from build123d import *

# Parameters (mm, degrees)
Y_KSEKLIK_EKSTR_ZYON1_DEPTH = 3.2
IZIM2_OUTSIDE_W             = 23.4
IZIM2_OUTSIDE_H             = 22.318
IZIM2_OUTSIDE_R             = 3.5
KES_EKSTR_ZYON1_DEPTH       = 3.2
KES_EKSTR_ZYON1_DRAFT       = -60
IZIM3_OUTSIDE_W             = 23.4
IZIM3_OUTSIDE_H             = 22.318
IZIM3_OUTSIDE_R             = 3.5
KES_EKSTR_ZYON2_DEPTH       = 3.2
KES_EKSTR_ZYON2_DRAFT       = -60
IZIM5_R                     = 1.545
KES_EKSTR_ZYON3_DEPTH       = 3.2
PAH1_SIZE                   = 0.65
KES_S_P_R1_PITCH            = 0.7
KES_S_P_R1_HEIGHT           = 4
KES_S_P_R1_RADIUS           = 1.545
BOSS_EXTRUDE1_DEPTH         = 3.21
BOSS_EXTRUDE1_DEPTH_BACK    = 0.01
SKETCH1_R                   = 3.5
SKETCH1_R_2                 = 2.2


with BuildPart() as part:
    # Çizim1 → Yükseklik-Ekstrüzyon1 (new body)
    with BuildSketch(Plane.XY):
        Polygon((4.041451884, 0), (2.020725942, 3.5), (-2.020725942, 3.5), (-4.041451884, 0), (-2.020725942, -3.5), (2.020725942, -3.5), align=None)
    extrude(amount=Y_KSEKLIK_EKSTR_ZYON1_DEPTH)


with BuildPart() as kes_ekstr_zyon1_tool:
    # Çizim2 outside → Kes-Ekstrüzyon1 (with draft: the straight prism first)
    with BuildSketch(Plane.XY.offset(3.2)):
        Rectangle(IZIM2_OUTSIDE_W, IZIM2_OUTSIDE_H)
        Circle(IZIM2_OUTSIDE_R, mode=Mode.SUBTRACT)
    extrude(amount=-KES_EKSTR_ZYON1_DEPTH)
    # Kes-Ekstrüzyon1: the draft: its side faces are tilted about the plane it starts from
    kes_ekstr_zyon1_sides = [kes_ekstr_zyon1_tool.faces().sort_by_distance(p)[0] for p in [
        (0, -11.159, 1.6),
        (11.7, 0, 1.6),
        (0, 11.159, 1.6),
        (-11.7, 0, 1.6),
        (-3.5, 0, 1.6),
    ]]
    draft(kes_ekstr_zyon1_sides, Plane.XY.offset(3.2), KES_EKSTR_ZYON1_DRAFT)


with BuildPart() as part_1:
    add(part.part)

    # Kes-Ekstrüzyon1: cut by kes_ekstr_zyon1_tool
    add(kes_ekstr_zyon1_tool.part, mode=Mode.SUBTRACT)


with BuildPart() as kes_ekstr_zyon2_tool:
    # Çizim3 outside → Kes-Ekstrüzyon2 (with draft: the straight prism first)
    with BuildSketch(Plane(origin=(0, 0, 0), x_dir=(-1, 0, 0), z_dir=(0, 0, -1))):
        Rectangle(IZIM3_OUTSIDE_W, IZIM3_OUTSIDE_H)
        Circle(IZIM3_OUTSIDE_R, mode=Mode.SUBTRACT)
    extrude(amount=-KES_EKSTR_ZYON2_DEPTH)
    # Kes-Ekstrüzyon2: the draft: its side faces are tilted about the plane it starts from
    kes_ekstr_zyon2_sides = [kes_ekstr_zyon2_tool.faces().sort_by_distance(p)[0] for p in [
        (0, -11.159, 1.6),
        (-11.7, 0, 1.6),
        (0, 11.159, 1.6),
        (11.7, 0, 1.6),
        (3.5, 0, 1.6),
    ]]
    draft(kes_ekstr_zyon2_sides, Plane(origin=(0, 0, 0), x_dir=(-1, 0, 0), z_dir=(0, 0, -1)), KES_EKSTR_ZYON2_DRAFT)


with BuildPart() as part_2:
    add(part_1.part)

    # Kes-Ekstrüzyon2: cut by kes_ekstr_zyon2_tool
    add(kes_ekstr_zyon2_tool.part, mode=Mode.SUBTRACT)

    # Çizim5 → Kes-Ekstrüzyon3 (cut)
    with BuildSketch(Plane(origin=(0, 0, 0), x_dir=(-1, 0, 0), z_dir=(0, 0, -1))):
        Circle(IZIM5_R)
    extrude(amount=-KES_EKSTR_ZYON3_DEPTH, mode=Mode.SUBTRACT)

    # Pah1
    pah1_edges = [part_2.edges().sort_by_distance(p)[0] for p in [
        (1.545, 0, 3.2),
        (1.545, 0, 0),
    ]]
    chamfer(pah1_edges, length=PAH1_SIZE)

    # Kes-Süpür1: sweep along a helix
    with BuildLine() as kes_s_p_r1_path:
        Helix(KES_S_P_R1_PITCH, KES_S_P_R1_HEIGHT, KES_S_P_R1_RADIUS, center=(0, 0, 0), direction=(0, 0, 1))
    # Çizim7 → Kes-Süpür1 (sweep, cut)
    with BuildSketch(Plane(origin=(-0.343794843, -1.506263624, 4), x_dir=(0.07011904852635167, -0.016004215256580363, -0.9974102386319182), z_dir=(0.9724030815382076, -0.22194465783789016, 0.07192229051010418))):
        Polygon((0.347294283, 0.146531344), (-0.347294283, 0.146531344), (0, -0.455), align=None)
    sweep(path=kes_s_p_r1_path.line, is_frenet=True, mode=Mode.SUBTRACT)

    # Sketch1 → Boss-Extrude1 (add, two sides: drawn at the far end of the back side and taken through both)
    with BuildSketch(Plane.XY.offset(-BOSS_EXTRUDE1_DEPTH_BACK)):
        Circle(SKETCH1_R)
        Circle(SKETCH1_R_2, mode=Mode.SUBTRACT)
    extrude(amount=BOSS_EXTRUDE1_DEPTH + BOSS_EXTRUDE1_DEPTH_BACK)


solid = part_2.part
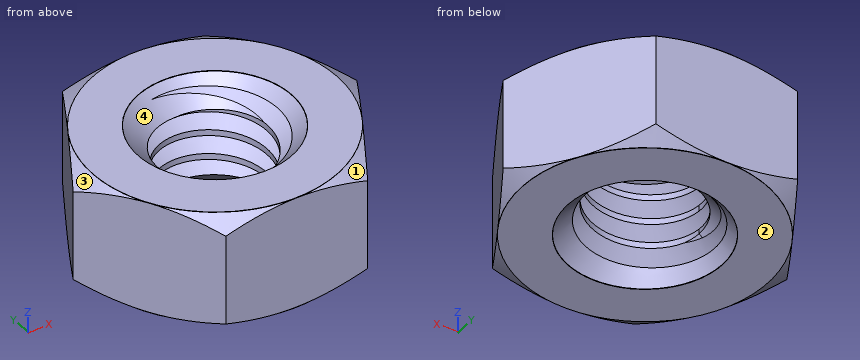
Verification items for the finished model (mm, model axes). Face numbers are marked on the shaded views. Coordinates: 2 decimals unless noted, no trailing zeros. One line per item, written item: value. Start each with the question number.
Q1. Thickness scan on L1, parallel to Y at x = 0, z = 1.1; L2, parallel to X at y = 0, z = 0.05 (3 decimals); L3, parallel to Y at x = 0, z = 1.05. Record the ranges inside material, lowest first. Write a range as from..to.
Q2. Go/stop test with flat-tipped pins: P1, Ø3.5, axis at x = 0, y = 0, coming from the -Z side (3 decimals); P2, Ø1, axis at y = 1.5, z = 0.5, coming from the -X side; P3, Ø3.5, axis at x = 0, y = 0, coming from the +Z side (3 decimals). Record where each tip stops, or that it passes through.
Q3. Cross-section at A-A on x = 1.75. State how many separate pieces and enclosed holes the cut face has, and give its area (3 significant figures).
Q4. Mould release check, pull along X, two halves, no side actions. Record for the marked faces 1, 2, 3 and 4: pulls with the +X half, pulls with the -X half, needs draft (parallel to the pull), parting line crosses it, or undercut.
Checked values:
1. L1: y = -3.5..-1.78, 1.61..3.5
1. L2: x = -3.587..-2.145, 2.145..3.587
1. L3: y = -3.5..-1.7, 1.7..3.5
2. P1: stops at z = 0.445
2. P2: stops at x = -3.46
2. P3: stops at z = 2.755
3. separate pieces: 1
3. enclosed holes: 3
3. area: 19.4 mm²
4. face 1: pulls with the +X half
4. face 2: needs draft
4. face 3: pulls with the -X half
4. face 4: undercut
